Source: CAD feature listing. Evaluate the final solid. Frame: model axes, mm. Face numbers are marked on the shaded views. A direction names the side the tool comes from. Round coordinates to 2 decimals unless told otherwise and drop trailing zeros. Write each loop counter-clockwise with the first axis right and the second up, starting at its lowest first coordinate (ties: lowest second). Pieces come first, ordered by that corner, then holes.
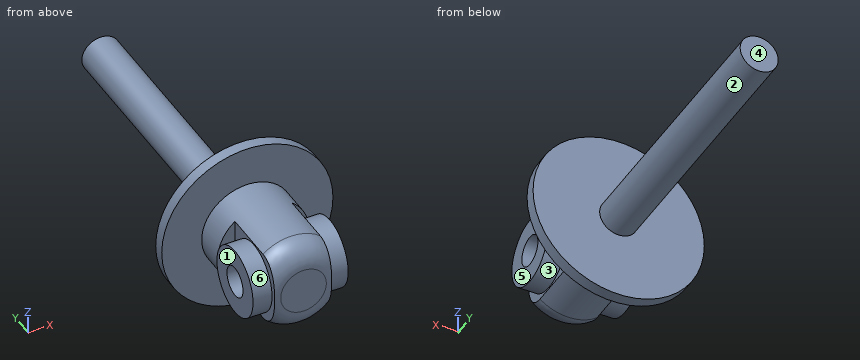
```python
from build123d import *

# Parameters (mm, degrees)
SKETCH1_R               = 225
BOSS_EXTRUDE1_DEPTH     = 30
SKETCH2_R               = 50
BOSS_EXTRUDE2_DEPTH     = 700
SKETCH3_R               = 120
BOSS_EXTRUDE3_DEPTH     = 280
FILLET1_R               = 60
SKETCH4_W               = 195.7
SKETCH4_H               = 200
CUT_EXTRUDE1_DEPTH      = 226
CUT_EXTRUDE1_DEPTH_BACK = 226
SKETCH5_R               = 40
CUT_EXTRUDE2_DEPTH      = 301
SKETCH6_R               = 90
SKETCH6_R_2             = 40
BOSS_EXTRUDE4_DEPTH     = 125
SCALE1_SCALE            = 0.4


with BuildPart() as part:
    # Sketch1 → Boss-Extrude1 (new body)
    with BuildSketch(Plane(origin=(0, 0, 0), x_dir=(1, 0, 0), z_dir=(0, 1, 0))):
        Circle(SKETCH1_R)
    extrude(amount=BOSS_EXTRUDE1_DEPTH)

    # Sketch2 → Boss-Extrude2 (add)
    with BuildSketch(Plane(origin=(0, 30, 0), x_dir=(1, 0, 0), z_dir=(0, 1, 0))):
        Circle(SKETCH2_R)
    extrude(amount=BOSS_EXTRUDE2_DEPTH)

    # Sketch3 → Boss-Extrude3 (add)
    with BuildSketch(Plane.XZ):
        Circle(SKETCH3_R)
    extrude(amount=BOSS_EXTRUDE3_DEPTH)

    # Fillet1
    fillet1_edges = [part.edges().sort_by_distance(p)[0] for p in [
        (-120, -280, 0),
    ]]
    fillet(fillet1_edges, radius=FILLET1_R)

    # Sketch4 → Cut-Extrude1 (cut, two sides)
    with BuildSketch(Plane.XY) as cut_extrude1_sk:
        with Locations((172.85, -180)):
            Rectangle(SKETCH4_W, SKETCH4_H)
        with Locations((-172.85, -180)):
            Rectangle(SKETCH4_W, SKETCH4_H)
    extrude(amount=CUT_EXTRUDE1_DEPTH, mode=Mode.SUBTRACT)
    extrude(cut_extrude1_sk.sketch, amount=-CUT_EXTRUDE1_DEPTH_BACK, mode=Mode.SUBTRACT)

    # Sketch5 → Cut-Extrude2 (cut, through all)
    with BuildSketch(Plane(origin=(75, 0, 0), x_dir=(0, 0, -1), z_dir=(1, 0, 0))):
        with Locations((0, -175.331172544)):
            Circle(SKETCH5_R)
    extrude(amount=-CUT_EXTRUDE2_DEPTH, mode=Mode.SUBTRACT)

    # Sketch6 → Boss-Extrude4 (add, symmetric)
    with BuildSketch(Plane(origin=(0, 0, 0), x_dir=(0, 0, -1), z_dir=(1, 0, 0))):
        with Locations((0, -175.331172544)):
            Circle(SKETCH6_R)
        with Locations((0, -175.331172544)):
            Circle(SKETCH6_R_2, mode=Mode.SUBTRACT)
    extrude(amount=BOSS_EXTRUDE4_DEPTH, both=True)


with BuildPart() as part_1:
    # Scale1: scaled about (-3.146e-06, 30.247926965, -1.0493e-05)
    add(part.part.scale(SCALE1_SCALE).moved(Location((-1.888e-06, 18.148756179, -6.296e-06))))


solid = part_1.part
```
Q1. Section query B-B, the plane y = 2. Output: boundary loops of the cut face in (x, z).
Q2. Section query A-A, the plane x = 37. Output: boundary loops of the cut face in (y, z), and give its area (3 significant figures).
Q3. Section query C-C, the plane z = 61. Output: boundary loops of the cut face in (x, y).
Q4. Line query: line 1 (X direction, y = -58, z = 37); line 2 (Y direction, x = -45, z = -71); line 3 (Y direction, x = -46, z = 25). Output: solid intervals per line, ascending.
Q5. Section query D-D, the plane x = 75. Output: boundary loops of the cut face in (y, z).
Q6. Pin query (flat end, axial travel): P1, Ø21.5, axis at y = -40, z = -6.5, coming from the -X side; P2, Ø22.5, axis at y = -63.5, z = -13, coming from the +X side; P3, Ø4, axis at x = 34, z = 65.5, coming from the +Y side. Return the tip coordinate at first contact, or that it passes through.
Q7. Set-up query: the marked faces 1, 2 and 3. Return all of +Z, -Z, +X, -X, +Y, -Y with unobstructed straight access to the full face (end or side cutting, diameter ignored); none if empty.
Q8. Mould query, pull axis Y, two halves, no side actions, for the marked faces 4, 5 and 6. Classes: pulls with the +Y half, pulls with the -Y half, needs draft (parallel to the pull), parting line crosses it, or undercut.
Filled in:
1. outline: circle Ø96 at (0, 0)
2. outline: circle Ø72 at (-51.98, 0); (-13.85, -30.58) - (18.15, -30.58) - (18.15, -82.04) - (30.15, -82.04) - (30.15, 82.04) - (18.15, 82.04) - (18.15, 30.58) - (-13.85, 30.58) - close; hole circle Ø32 at (-51.98, 0)
2. area: 7,190 mm2
3. outline: (-66.17, 18.15) - (66.17, 18.15) - (66.17, 30.15) - (-66.17, 30.15) - close
4. line 1: x = -30 to 30
4. line 2: y = 18.15 to 30.15
4. line 3: y = -77.89 to -26.08, 18.15 to 30.15
5. outline: (18.15, -49.75) - (30.15, -49.75) - (30.15, 49.75) - (18.15, 49.75) - close
6. P1: stops at x = -50
6. P2: stops at x = 50
6. P3: stops at y = 30.15
7. face 1: +Z, -Z, -X, -Y
7. face 2: +Y
7. face 3: +X
8. face 4: pulls with the +Y half
8. face 5: needs draft
8. face 6: undercut
